```python
from build123d import *

# Parameters (mm, degrees)
F1_DEPTH = 5
F3_DEPTH = 2.5
F4_SIZE  = 5
F5_SIZE  = 0.5


with BuildPart() as f1:
    # F0 (on Top) → F1 (new body)
    with BuildSketch(Plane.XY):
        with BuildLine():
            Line((-9, 0), (0, 0))
            Line((0, 0), (0, 106.5))
            Line((0, 106.5), (-9, 106.5))
            Line((-9, 106.5), (-9, 103.5))
            ThreePointArc((-9, 103.5), (-7.585786, 102.914214), (-7, 101.5))
            ThreePointArc((-7, 101.5), (-7.585786, 100.085786), (-9, 99.5))
            Line((-9, 99.5), (-9, 96.5))
            Line((-9, 96.5), (-9, 80))
            Line((-9, 80), (-9, 77))
            ThreePointArc((-9, 77), (-7.585786, 76.414214), (-7, 75))
            ThreePointArc((-7, 75), (-7.585786, 73.585786), (-9, 73))
            Line((-9, 73), (-9, 70))
            Line((-9, 70), (-9, 10))
            Line((-9, 10), (-9, 7))
            ThreePointArc((-9, 7), (-7.585786, 6.414214), (-7, 5))
            ThreePointArc((-7, 5), (-7.585786, 3.585786), (-9, 3))
            Line((-9, 3), (-9, 0))
        make_face()
        with BuildLine():
            ThreePointArc((-9, 10), (-14, 5), (-9, 0))
            Line((-9, 0), (-9, 3))
            ThreePointArc((-9, 3), (-11, 5), (-9, 7))
            Line((-9, 7), (-9, 10))
        make_face()
        with BuildLine():
            Line((-9, 103.5), (-9, 106.5))
            ThreePointArc((-9, 106.5), (-14, 101.5), (-9, 96.5))
            Line((-9, 96.5), (-9, 99.5))
            ThreePointArc((-9, 99.5), (-11, 101.5), (-9, 103.5))
        make_face()
        with BuildLine():
            ThreePointArc((-9, 80), (-14, 75), (-9, 70))
            Line((-9, 70), (-9, 73))
            ThreePointArc((-9, 73), (-11, 75), (-9, 77))
            Line((-9, 77), (-9, 80))
        make_face()
    extrude(amount=F1_DEPTH)

    # F2 (on face) → F3 (cut)
    with BuildSketch(Plane(origin=(0, 0, 0), x_dir=(1, 0, 0), z_dir=(0, 0, -1))):
        with BuildLine():
            Line((0, -96.5), (-9, -96.5))
            ThreePointArc((-9, -96.5), (-14, -101.5), (-9, -106.5))
            Line((-9, -106.5), (0, -106.5))
            Line((0, -106.5), (0, -96.5))
        make_face()
    extrude(amount=-F3_DEPTH, mode=Mode.SUBTRACT)

    # F4
    f4_edges = [f1.edges().sort_by_distance(p)[0] for p in [
        (0, 0, 2.5),
    ]]
    chamfer(f4_edges, length=F4_SIZE)

    # F5
    f5_edges = [f1.edges().sort_by_distance(p)[0] for p in [
        (-7, 0, 5),
        (-2.5, 2.5, 5),
        (-14, 5, 5),
        (0, 55.75, 5),
        (-9, 40, 5),
        (-4.5, 106.5, 5),
        (-14, 75, 5),
        (-14, 101.5, 5),
        (-9, 88.25, 5),
        (-9, 73, 5),
        (-9, 99.5, 5),
        (-9, 3, 5),
        (0, 50.75, 0),
        (-2.5, 2.5, 0),
        (-4.5, 96.5, 0),
        (-7, 0, 0),
        (-9, 88.25, 0),
        (-14, 5, 0),
        (-14, 75, 0),
        (-9, 40, 0),
        (-9, 3, 0),
        (-9, 73, 0),
    ]]
    chamfer(f5_edges, length=F5_SIZE)


solid = f1.part
```
CAD build for the part. Positions are in the model's coordinates, mm. A direction names the side the tool comes from. Round coordinates to 2 decimals unless told otherwise and drop trailing zeros. Write each loop counter-clockwise with the first axis right and the second up, starting at its lowest first coordinate (ties: lowest second). Pieces come first, ordered by that corner, then holes. Notation, with made-up numbers: (10, -18) - (41, -18) arc R12 cw to (41, -4) - close; hole circle Ø10 at (36.5, 74.5). An arc over 180 degrees is marked (long way). Return JSON: item names as keys, results as strings. Group by question number.
Item 1: 3-axis set-ups, long thin cutter, end or side, ignore diameter. For faces 1 (the face through (-4, 96.5, 1)), 2 (the face through (-9, 40, 2)), 3 (the face through (0, 55, 2)): which of +Z, -Z, +X, -X, +Y, -Y reach the whole face in a straight line?
Item 2: Band-saw the part on A-A on y = 42. List the corners of the cut face in (x, z).
Item 3: Band-saw the part on B-B on x = -1.75. List the corners of the cut face in (y, z), plus the area to 3 significant figures.
Item 4: Probe probe 1 along Y at (x, z) = (-8.75, 4.2); probe 2 along Y at (x, z) = (-10.5, 3.65); probe 3 along Y at (x, z) = (-7.75, 0.6). List the from-to ranges inside material, lowest first.
Item 5: Mould opens along Y. For faces 4 (the face through (-13.64, 75.11, 4.86)), 5 (the face through (-2.71, 2.64, 0.25)), 6 (the face through (-6, 101, 2.5)) say: +Y half, -Y half, draft (parallel to the pull), parting line (faces both ways), or undercut.
Item 6: Flat gauge pins, fed straight in: pin 1 Ø8 at (x, y) = (-9, 101) entering from -Z; pin 2 Ø3 at (y, z) = (73, 1) entering from -X; pin 3 Ø3 at (y, z) = (27, 3) entering from -X; pin 4 Ø2 at (x, z) = (-5, 2) entering from +Y. Where does each tip first touch, or does it go through?
Resolved:
{
 "1": {"face 1": "-Z, +X, -X, +Y", "face 2": "+Z, -Z, -X", "face 3": "+Z, -Z, +X, +Y, -Y"},
 "2": {"outline": "(-9, 0.5) - (-8.5, 0) - (-0.5, 0) - (0, 0.5) - (0, 4.5) - (-0.5, 5) - (-8.5, 5) - (-9, 4.5) - close"},
 "3": {"outline": "(3.25, 0.5) - (3.96, 0) - (96, 0) - (96.5, 0.5) - (96.5, 2.5) - (106.5, 2.5) - (106.5, 4.5) - (106, 5) - (3.96, 5) - (3.25, 4.5) - close", "area": "491 mm²"},
 "4": {"probe 1": "y = 0 to 3.02, 6.98 to 73.02, 76.98 to 99.52, 103.48 to 106.5", "probe 2": "y = 0.23 to 3.68, 6.32 to 9.77, 70.23 to 73.68, 76.32 to 79.77, 96.73 to 100.18, 102.82 to 106.27", "probe 3": "y = 0 to 3.44, 6.56 to 73.44, 76.56 to 96.5"},
 "5": {"face 4": "undercut", "face 5": "-Y half", "face 6": "draft"},
 "6": {"pin 1": "stops at z = 2.5", "pin 2": "stops at x = -13.97", "pin 3": "stops at x = -9", "pin 4": "stops at y = 106.5"}
}
